Read the model definition and answer for the solid it produces. Units are mm, in the model's axes. A direction names the side the tool comes from. Give positions to 0.01 mm unless a question says otherwise; leave off trailing zeros. Order: outer loops, then holes, each group sorted by start corner. A loop starts at its lowest first (then second) coordinate and runs counter-clockwise, first axis right, second up. Notation, with made-up numbers: (58.25, 77) -> (84.25, 77) arc R30 ccw to (84.25, 107) -> close; hole circle Ø10 at (-34, -37). An arc over 180 degrees is marked (long way). One line per question, with ' | ' between items. Start each with the question number.
```python
from build123d import *

# Parameters (mm, degrees)
F0_R     = 3.96875
F0_R_2   = 2.8575
F1_DEPTH = 4.826
F2_DEPTH = 2.413


with BuildPart() as f1:
    # F0 (on Top) → F1 (new body)
    with BuildSketch(Plane.XY):
        Circle(F0_R)
        Circle(F0_R_2, mode=Mode.SUBTRACT)
    extrude(amount=F1_DEPTH)

    # F0 (on Top) → F2 (join)
    with BuildSketch(Plane.XY):
        with BuildLine():
            ThreePointArc((5.649248, 7.107538), (0.129327, 12.699882), (-5.463016, 7.179962))
            Line((-5.463016, 7.179962), (-5.556132, -7.107235))
            ThreePointArc((-5.556132, -7.107235), (-0.036212, -12.699579), (5.556132, -7.179658))
            Line((5.556132, -7.179658), (5.649248, 7.107538))
        make_face()
        Circle(F0_R, mode=Mode.SUBTRACT)
    extrude(amount=F2_DEPTH)


solid = f1.part
```
Q1. A cutting plane is placed at C-C, the plane z = 0.7. Determine the outline of the cut face in (x, y) (1 decimal), then the cut area to 3 significant figures.
Q2. A cutting plane is placed at A-A, the plane y = 1.25. Determine the outline of the cut face in (x, z), then the cut area to 3 significant figures.
Q3. A cutting plane is placed at B-B, the plane x = 1.5. Determine the outline of the cut face in (y, z), then the cut area to 3 significant figures.
Q4. A cutting plane is placed at D-D, the plane x = -3.5. Determine the outline of the cut face in (y, z).
Q5. Find the intervals of material crossed by line 1 (Y direction, x = 0, z = 3.5); line 2 (Z direction, x = 2.25, y = -11.25); line 3 (Y direction, x = 0, z = 1.9), in increasing order.
Q6. Which of the six approach directions +Z, -Z, +X, -X, +Y, -Y give full straight-line access (tool end or side, diameter ignored) to faces 4 (the flat face through (-1, 3, 4.826)), 5 (the cylindrical face through (-0.86, -3.874, 3.603))?
Q7. Determine the mould class of faces 1 (the cylindrical face through (0.251, 12.698, 1.19)), 2 (the flat face through (4, -3, 2.413)), 3 (the cylindrical face through (2.726, 0.858, 2.379)) for opening direction X: pulls with the +X half, pulls with the -X half, needs draft (parallel to the pull), parting line crosses it, or undercut.
Geometry results:
1) outline: (-5.6, -7.1) arc R5.6 ccw to (5.6, -7.2) -> (5.6, 7.1) arc R5.6 ccw to (-5.5, 7.2) -> close; hole circle Ø5.7 at (0, 0) | area: 230 mm²
2) outline: (-5.5, 0) -> (-2.57, 0) -> (-2.57, 4.83) -> (-3.77, 4.83) -> (-3.77, 2.41) -> (-5.5, 2.41) -> close; (2.57, 0) -> (5.61, 0) -> (5.61, 2.41) -> (3.77, 2.41) -> (3.77, 4.83) -> (2.57, 4.83) -> close | area: 20.2 mm²
3) outline: (-12.49, 0) -> (-2.43, 0) -> (-2.43, 4.83) -> (-3.67, 4.83) -> (-3.67, 2.41) -> (-12.49, 2.41) -> close; (2.43, 0) -> (12.52, 0) -> (12.52, 2.41) -> (3.67, 2.41) -> (3.67, 4.83) -> (2.43, 4.83) -> close | area: 54.6 mm²
4) outline: (-11.46, 0) -> (11.38, 0) -> (11.38, 2.41) -> (1.87, 2.41) -> (1.87, 4.83) -> (-1.87, 4.83) -> (-1.87, 2.41) -> (-11.46, 2.41) -> close
5) line 1: -3.97 to -2.86, 2.86 to 3.97 | line 2: 0 to 2.41 | line 3: -12.7 to -2.86, 2.86 to 12.7
6) face 4: +Z, +X, -X, +Y, -Y | face 5: +Z
7) face 1: parting line crosses it | face 2: needs draft | face 3: undercut
